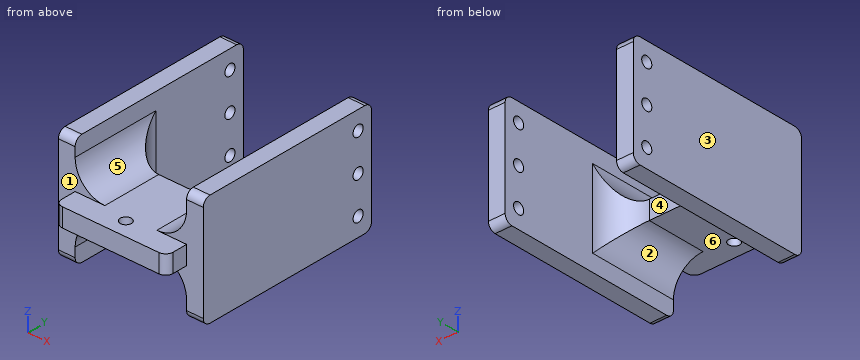
from build123d import *

# Parameters (mm, degrees)
SKETCH_1_W          = 30
SKETCH_1_H          = 50
EXTRUDE_1_DEPTH     = 5
SKETCH_5_W          = 30
SKETCH_5_H          = 50
EXTRUDE_2_DEPTH     = 4.5
SKETCH_6_R          = 1.5
CUT_EXTRUDE_1_DEPTH = 73.857738093
SKETCH_7_R          = 1.5
CUT_EXTRUDE_2_DEPTH = 73.857738093
SKETCH_10_R         = 1.5
CUT_EXTRUDE_3_DEPTH = 65.556177086
SKETCH_11_W         = 30
SKETCH_11_H         = 28
CUT_EXTRUDE_4_DEPTH = 65.556177086
FILLET_1_R          = 8
FILLET_2_R          = 8
FILLET_3_R          = 2


with BuildPart() as part:
    # 草图1 → 凸台-拉伸1 (new body)
    with BuildSketch(Plane.XY):
        Rectangle(SKETCH_1_W, SKETCH_1_H)
    extrude(amount=EXTRUDE_1_DEPTH)

    # 草图5 → 凸台-拉伸2 (add)
    with BuildSketch(Plane.ZY.offset(15)):
        with Locations((2.5, 34)):
            Rectangle(SKETCH_5_W, SKETCH_5_H)
    extrude_2 = extrude(amount=EXTRUDE_2_DEPTH)

    # 镜向1: 凸台-拉伸2 across plane
    add(extrude_2.mirror(Plane(origin=(0, 0, 0), x_dir=(0, 0, 1), z_dir=(1, 0, 0))))

    # 草图6 → 切除-拉伸1 (cut, through all)
    with BuildSketch(Plane.ZY.offset(19.5)):
        with Locations((2.5, 55)):
            Circle(SKETCH_6_R)
    extrude(amount=-CUT_EXTRUDE_1_DEPTH, mode=Mode.SUBTRACT)

    # 草图7 → 切除-拉伸2 (cut, through all)
    with BuildSketch(Plane.ZY.offset(19.5)):
        with Locations((-7.5, 55)):
            Circle(SKETCH_7_R)
        with Locations((12.5, 55)):
            Circle(SKETCH_7_R)
    extrude(amount=-CUT_EXTRUDE_2_DEPTH, mode=Mode.SUBTRACT)

    # 草图10 → 切除-拉伸3 (cut, through all)
    with BuildSketch(Plane(origin=(0, 0, 0), x_dir=(-1, 0, 0), z_dir=(0, 0, -1))):
        with Locations((0, -13.5)):
            Circle(SKETCH_10_R)
        with Locations((0, 7.5)):
            Circle(SKETCH_10_R)
    extrude(amount=-CUT_EXTRUDE_3_DEPTH, mode=Mode.SUBTRACT)

    # 草图11 → 切除-拉伸4 (cut, through all)
    with BuildSketch(Plane(origin=(0, 0, 0), x_dir=(-1, 0, 0), z_dir=(0, 0, -1))):
        with Locations((0, -11)):
            Rectangle(SKETCH_11_W, SKETCH_11_H)
    extrude(amount=-CUT_EXTRUDE_4_DEPTH, mode=Mode.SUBTRACT)

    # 圆角1
    fillet_1_edges = [part.edges().sort_by_distance(p)[0] for p in [
        (15, 17, 0),
        (15, 17, 5),
        (-15, 17, 5),
        (-15, 17, 0),
    ]]
    fillet(fillet_1_edges, radius=FILLET_1_R)

    # 圆角2
    fillet_2_edges = [part.edges().sort_by_distance(p)[0] for p in [
        (-15, 25, 2.5),
        (15, 25, 2.5),
    ]]
    fillet(fillet_2_edges, radius=FILLET_2_R)

    # 圆角3
    fillet_3_edges = [part.edges().sort_by_distance(p)[0] for p in [
        (-15, 3, 2.5),
        (15, 3, 2.5),
        (-17.25, 59, -12.5),
        (-17.25, 9, -12.5),
        (-17.25, 9, 17.5),
        (-17.25, 59, 17.5),
        (17.25, 9, -12.5),
        (17.25, 59, -12.5),
        (17.25, 59, 17.5),
        (17.25, 9, 17.5),
    ]]
    fillet(fillet_3_edges, radius=FILLET_3_R)


solid = part.part
Design review of the part built by this model. Coordinates are the model's own, in mm. Face numbers are marked on the shaded views. A direction names the side the tool comes from. Round coordinates to 2 decimals unless told otherwise and drop trailing zeros. Order: outer loops, then holes, each group sorted by start corner. A loop starts at its lowest first (then second) coordinate and runs counter-clockwise, first axis right, second up.
1) Consider section D-D (y = 39.5). State the section outline as (x, z) points.
The answers:
outline: (-19.5, -12.5) - (-15, -12.5) - (-15, 17.5) - (-19.5, 17.5) - close; (15, -12.5) - (19.5, -12.5) - (19.5, 17.5) - (15, 17.5) - close
2) Consider section A-A (y = 55). Count the separate pieces of the cut face and the enclosed holes in it, plus the area to 3 significant figures.
The answers:
separate pieces: 8
enclosed holes: 0
area: 189 mm2
3) Consider section B-B (x = 0). State the section outline as (y, z) points.
The answers:
outline: (3, 0) - (6, 0) - (6, 5) - (3, 5) - close; (9, 0) - (25, 0) - (25, 5) - (9, 5) - close
4) Machinability: for the marked faces 4, 5 and 6, which of the approach directions +Z, -Z, +X, -X, +Y, -Y give a long, thin tool a straight path to every point of the face, cutting with its end or side? Answer none if there is none.
The answers:
face 4: +Z, -Z, +Y
face 5: +Z, +Y, -Y
face 6: -Z, -Y
5) Consider section C-C (z = 2.5). State the section outline as (x, y) points, plus the area to 3 significant figures.
The answers:
outline: (-19.5, 9) - (-15, 9) - (-15, 5) arc R2 ccw to (-13, 3) - (13, 3) arc R2 ccw to (15, 5) - (15, 9) - (19.5, 9) - (19.5, 53.5) - (15, 53.5) - (15, 33) arc R8 cw to (7, 25) - (-7, 25) arc R8 cw to (-15, 33) - (-15, 53.5) - (-19.5, 53.5) - close; (-19.5, 56.5) - (-15, 56.5) - (-15, 59) - (-19.5, 59) - close; (15, 56.5) - (19.5, 56.5) - (19.5, 59) - (15, 59) - close; hole circle Ø3 at (0, 7.5)
area: 1,100 mm2
6) Draft analysis for pull direction X (two halves, no side actions). For the marked faces 1, 2 and 3, state which applies: released by +X, released by -X, zero draft, split by the parting line, or undercut.
The answers:
face 1: zero draft
face 2: undercut
face 3: released by -X
7) For L1, parallel to X at y = 37.5, z = 15.25; L2, parallel to Y at x = -17.1, z = -7.5; L3, parallel to X at y = 12, z = 6.25, list the stretches that pass through material, from the lowest coordinate up.
The answers:
L1: x = -19.5 to -15, 15 to 19.5
L2: y = 9 to 53.5, 56.5 to 59
L3: x = -19.5 to -11.29, 11.29 to 19.5
8) Clearance check with flat-ended pins moving along their axes: pin 1 Ø2.5 at (x, z) = (0.5, 3.5) entering from +Y; pin 2 Ø17.5 at (x, y) = (2, 14.5) entering from -Z; pin 3 Ø4 at (x, y) = (0, 7.5) entering from +Z. State where each tip first meets the part, or that it passes through.
The answers:
pin 1: stops at y = 25
pin 2: stops at z = -0.93
pin 3: stops at z = 5
